Here's the drawing with two shaded views (mm, measured from the low corner). I have some questions. A direction names the side the tool comes from. Round coordinates to 2 decimals unless told otherwise and drop trailing zeros. Order: outer loops, then holes, each group sorted by start corner. A loop starts at its lowest first (then second) coordinate and runs counter-clockwise, first axis right, second up.
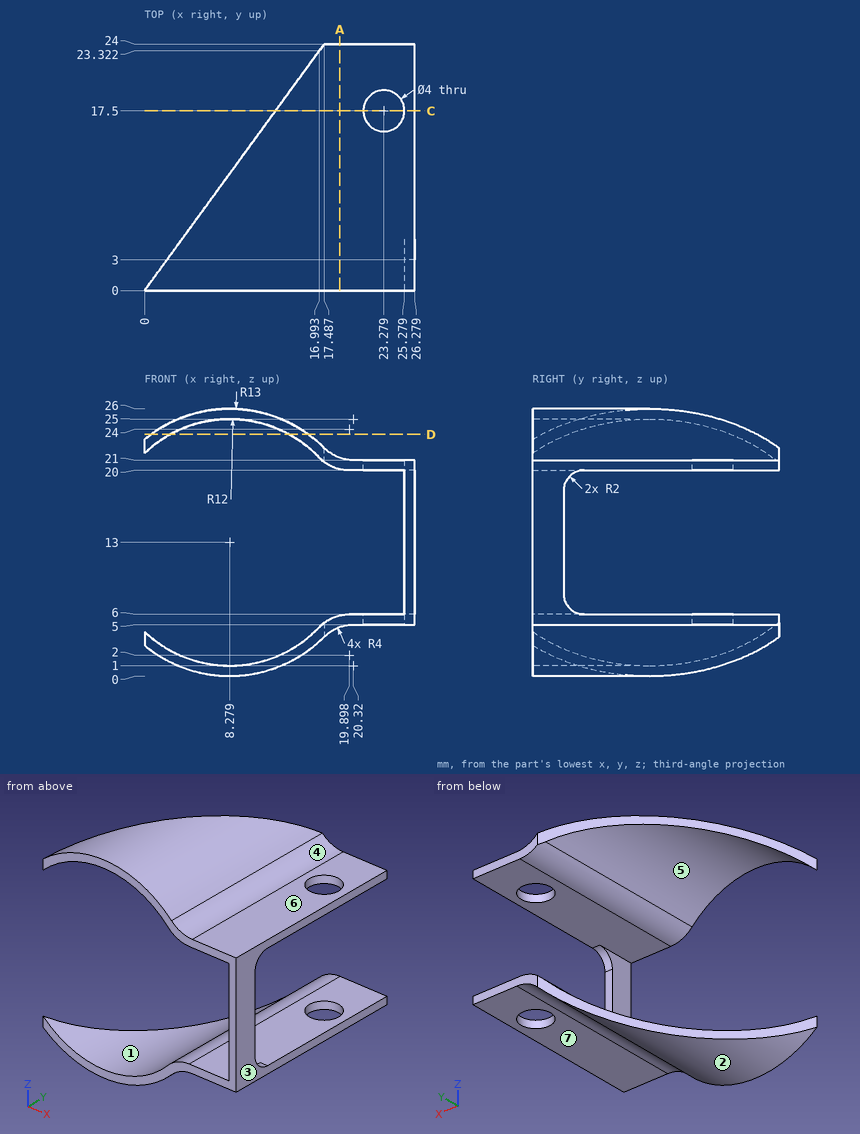
1. If we section it at D-D, the plane z = 23.5: Write out the boundary of the cut face in (x, y) (1 decimal).
Evaluation:
outline: (0.6, 0) - (2.5, 0) - (2.5, 3.4) - (0.6, 0.8) - close; (14.1, 0) - (15.9, 0) - (15.9, 21.9) - (14.1, 19.3) - close
2. I'm going to push flat-ended pins straight in: P1, Ø4.5, axis at x = 23.28, y = 17.5, coming from the +Z side; P2, Ø12, axis at x = 22.5, y = 19.5, coming from the +Z side; P3, Ø1.8, axis at x = 24, y = 7.5, coming from the -Z side. Where does each tip first touch, or does it pass through?
Evaluation:
P1: stops at z = 21
P2: stops at z = 23.07
P3: stops at z = 5
3. If we section it at A-A, the plane x = 19: Write out the boundary of the cut face in (y, z).
Evaluation:
outline: (0, 4.78) - (24, 4.78) - (24, 5.9) - (0, 5.9) - close; (0, 20.1) - (24, 20.1) - (24, 21.22) - (0, 21.22) - close
4. If we mould it in two halves opening along Z, with no side actions, what happens to the marked faces 1, 2, 3 and 4? For each: released by +Z, released by -Z, zero draft, split by the parting line, or undercut.
Evaluation:
face 1: undercut
face 2: released by -Z
face 3: zero draft
face 4: released by +Z
5. If we section it at C-C, the plane y = 17.5: State how many separate pieces and enclosed holes the cut face has.
Evaluation:
separate pieces: 4
enclosed holes: 0
6. I need wall thicknesses on probe 1 along Z at (x, y) = (24.75, 11.25); probe 2 along Z at (x, y) = (12.25, 2) (1 decimal); probe 3 along Y at (x, z) = (1.75, 2.25). Which ranges of each line are inside material? Lowest first, please.
Evaluation:
probe 1: z = 5 to 6, 20 to 21
probe 2: z = 0.6 to 1.7, 24.3 to 25.4
probe 3: y = 0 to 2.4
7. On a 3-axis mill with a long thin cutter (end or side, diameter ignored), from which of +Z, -Z, +X, -X, +Y, -Y can I reach the whole of each face in a straight line? I mean the marked faces 5, 6 and 7. Say none if no direction works.
Evaluation:
face 5: +Y, -Y
face 6: +Z, +X, +Y, -Y
face 7: -Z, +X, +Y, -Y
